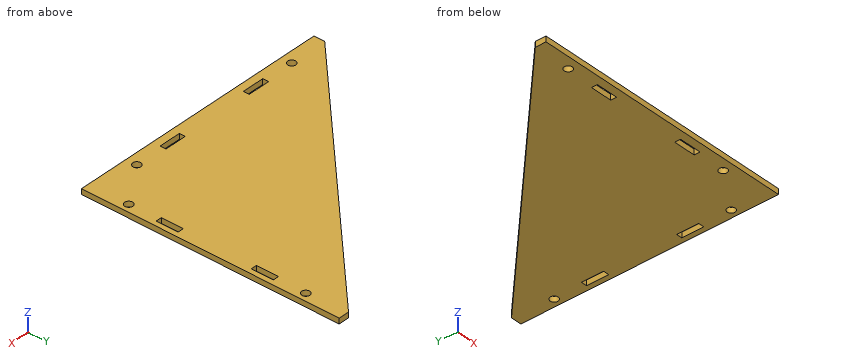
from build123d import *

# Parameters (mm, degrees)
SKETCH_1_R      = 1.5
SKETCH_1_W      = 8.2
SKETCH_1_H      = 2.2
SKETCH_1_W_2    = 2.2
SKETCH_1_H_2    = 8.2
EXTRUDE_1_DEPTH = 2


with BuildPart() as part:
    # 草图1 → 凸台-拉伸1 (new body)
    with BuildSketch(Plane.XY):
        Polygon((44.733844386, -118.574512395), (48.733844386, -118.574512395), (49.733844386, -118.574512395), (49.733844386, -22.574512395), (45.733844386, -22.574512395), (-49.266155614, -114.574512396), (-49.266155614, -118.574512395), (-3.266155614, -118.574512395), align=None)
        with Locations((-35.266155614, -114.574512396)):
            Circle(SKETCH_1_R, mode=Mode.SUBTRACT)
        with Locations(Location((30.733844386, -114.574512396, 0), (0, 0, 180))):
            Circle(SKETCH_1_R, mode=Mode.SUBTRACT)
        with Locations((46.733844387, -103.574512395)):
            Circle(SKETCH_1_R, mode=Mode.SUBTRACT)
        with Locations(Location((46.733844387, -37.616179062, 0), (0, 0, 180))):
            Circle(SKETCH_1_R, mode=Mode.SUBTRACT)
        with Locations((-20.016155614, -114.574512396)):
            Rectangle(SKETCH_1_W, SKETCH_1_H, mode=Mode.SUBTRACT)
        with Locations((15.483844386, -114.574512396)):
            Rectangle(SKETCH_1_W, SKETCH_1_H, mode=Mode.SUBTRACT)
        with Locations((46.733844387, -88.324512395)):
            Rectangle(SKETCH_1_W_2, SKETCH_1_H_2, mode=Mode.SUBTRACT)
        with Locations((46.733844387, -52.866179062)):
            Rectangle(SKETCH_1_W_2, SKETCH_1_H_2, mode=Mode.SUBTRACT)
    extrude(amount=EXTRUDE_1_DEPTH)


solid = part.part
Design review of the part built by this model. Coordinates are the model's own, in mm. Coordinates: 2 decimals unless noted, no trailing zeros. Order: outer loops, then holes, each group sorted by start corner. A loop starts at its lowest first (then second) coordinate and runs counter-clockwise, first axis right, second up.
Item 1: Take a section at D-D, the plane y = -35. Write out the cut boundary in (x, z).
Item 2: Take a section at A-A, the plane y = -91. Write out the cut boundary in (x, z).
Item 3: Take a section at B-B, the plane x = -23. Write out the cut boundary in (y, z), then the cut area to 3 significant figures.
Item 4: Take a section at C-C, the plane z = 0.85. Count the separate pieces of the cut face and the enclosed holes in it, then the cut area to 3 significant figures.
Item 5: For pin 1 Ø2.5 at (x, y) = (30.73, -114.57) entering from +Z; pin 2 Ø1 at (y, z) = (-53, 1.5) entering from -X; pin 3 Ø0.6 at (x, z) = (15, 1) entering from +Y, all flat-tipped, find the tip position at first contact; note any pin that passes through.
Item 6: For line 1 (Y direction, x = 32, z = 1.7); line 2 (Y direction, x = -22, z = 1.3); line 3 (X direction, y = -54.5, z = 0.8), list the stretches that pass through material, from the lowest coordinate up.
The answers:
1. outline: (32.9, 0) - (49.73, 0) - (49.73, 2) - (32.9, 2) - close
2. outline: (-24.92, 0) - (45.63, 0) - (45.63, 2) - (-24.92, 2) - close; (47.83, 0) - (49.73, 0) - (49.73, 2) - (47.83, 2) - close
3. outline: (-118.57, 0) - (-115.67, 0) - (-115.67, 2) - (-118.57, 2) - close; (-113.47, 0) - (-89.14, 0) - (-89.14, 2) - (-113.47, 2) - close
3. area: 54.5 mm2
4. separate pieces: 1
4. enclosed holes: 8
4. area: 5,030 mm2
5. pin 1: passes through
5. pin 2: stops at x = 13.8
5. pin 3: stops at y = -52.05
6. line 1: y = -118.57 to -115.38, -113.77 to -35.87
6. line 2: y = -118.57 to -115.67, -113.47 to -88.17
6. line 3: x = 12.77 to 45.63, 47.83 to 49.73
